Print and shaded views of the part. All mm, measured from the part's lowest x, y and z. Round coordinates to 2 decimals unless told otherwise and drop trailing zeros. Write each loop counter-clockwise with the first axis right and the second up, starting at its lowest first coordinate (ties: lowest second). Pieces come first, ordered by that corner, then holes.
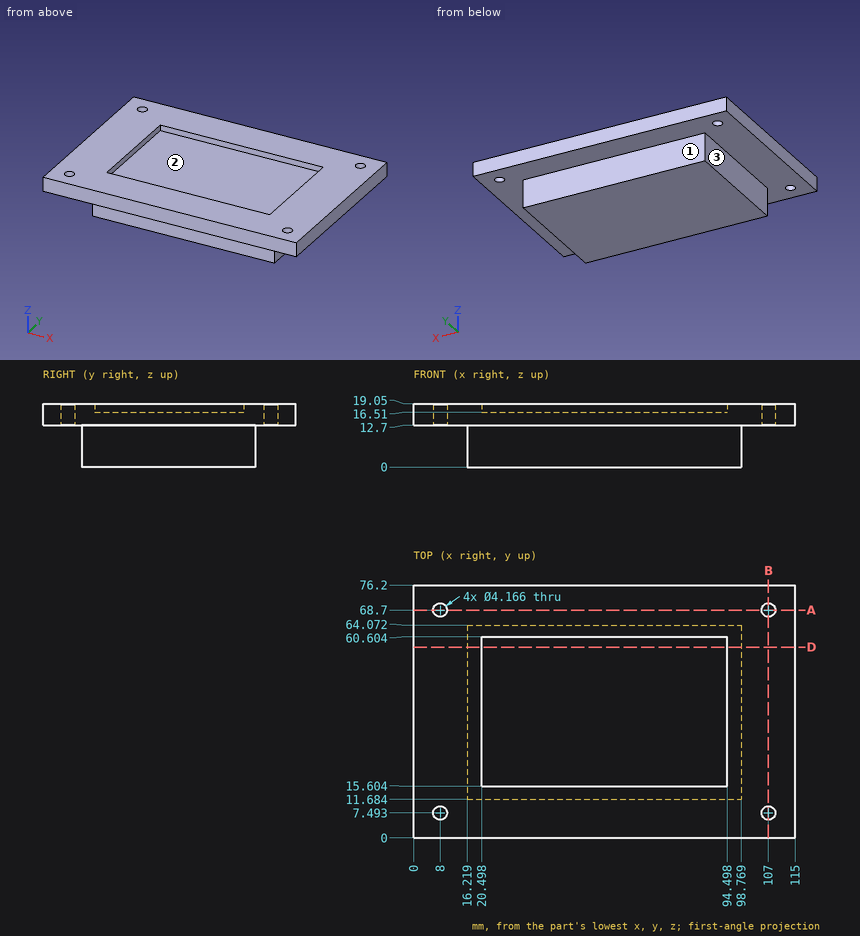
1) Slice it at A-A (y = 68.7). Write the cut outline in (x, z).
Results:
outline: (0, 12.7) - (5.92, 12.7) - (5.92, 19.05) - (0, 19.05) - close; (10.08, 12.7) - (104.92, 12.7) - (104.92, 19.05) - (10.08, 19.05) - close; (109.08, 12.7) - (115, 12.7) - (115, 19.05) - (109.08, 19.05) - close
2) Pin check, flat tips, straight feed: pin 1 Ø6.5 at (x, y) = (107, 68.7) entering from +Z; pin 2 Ø2 at (x, z) = (85.5, 10) entering from +Y; pin 3 Ø3 at (x, y) = (60.5, 66.5) entering from -Z; pin 4 Ø1.5 at (y, z) = (15, 9.5) entering from +X. Stop position of each tip, or through.
Results:
pin 1: stops at z = 19.05
pin 2: stops at y = 64.07
pin 3: stops at z = 12.7
pin 4: stops at x = 98.77
3) Slice it at D-D (y = 57.5). Write the cut outline in (x, z), plus the area to 3 significant figures.
Results:
outline: (0, 12.7) - (16.22, 12.7) - (16.22, 0) - (98.77, 0) - (98.77, 12.7) - (115, 12.7) - (115, 19.05) - (94.5, 19.05) - (94.5, 16.51) - (20.5, 16.51) - (20.5, 19.05) - (0, 19.05) - close
area: 1,590 mm2
4) Mould opens along Y. For the marked faces 1, 2 and 3 say: released by +Y, released by -Y, zero draft, split by the parting line, or undercut.
Results:
face 1: released by +Y
face 2: undercut
face 3: zero draft
5) Wall check: L1, parallel to Y at x = 107, z = 15.25 (1 decimal); L2, parallel to Y at x = 72, z = 17.75 (1 decimal); L3, parallel to X at y = 55.5, z = 18. Give the ranges that are in metal, low to high.
Results:
L1: y = 0 to 5.4, 9.6 to 66.6, 70.8 to 76.2
L2: y = 0 to 15.6, 60.6 to 76.2
L3: x = 0 to 20.5, 94.5 to 115
6) Slice it at B-B (x = 107). Count the separate pieces of the cut face and the enclosed holes in it, plus the area to 3 significant figures.
Results:
separate pieces: 3
enclosed holes: 0
area: 431 mm2
